from build123d import *

# Parameters (mm, degrees)
F1_DEPTH = 20
F2_R     = 5
F4_DEPTH = 8
F5_R     = 5
F6_DEPTH = 8


with BuildPart() as f1:
    # F0 (on Front) → F1 (new body, symmetric)
    with BuildSketch(Plane.XZ):
        with BuildLine():
            Line((-40, -35), (-32, -35))
            Line((-32, -35), (-32, 22))
            ThreePointArc((-32, 22), (-30.535534, 25.535534), (-27, 27))
            Line((-27, 27), (40, 27))
            Line((40, 27), (40, 35))
            Line((40, 35), (-27, 35))
            ThreePointArc((-27, 35), (-36.192388, 31.192388), (-40, 22))
            Line((-40, 22), (-40, -35))
        make_face()
    extrude(amount=F1_DEPTH, both=True)

    # F2
    f2_edges = [f1.edges().sort_by_distance(p)[0] for p in [
        (40, -20, 31),
        (40, 20, 31),
        (-36, -20, -35),
        (-36, 20, -35),
    ]]
    fillet(f2_edges, radius=F2_R)

    # F3 (on face) → F4 (cut, through all)
    with BuildSketch(Plane.XY.offset(35)):
        with BuildLine():
            Line((8, -4), (20, -4))
            ThreePointArc((20, -4), (24, 0), (20, 4))
            Line((20, 4), (8, 4))
            ThreePointArc((8, 4), (4, 0), (8, -4))
        make_face()
    extrude(amount=-F4_DEPTH, mode=Mode.SUBTRACT)

    # F5 (on face) → F6 (cut, through all)
    with BuildSketch(Plane.YZ.offset(-32)):
        with Locations((0, -20)):
            Circle(F5_R)
        with Locations((0, 5)):
            Circle(F5_R)
    extrude(amount=-F6_DEPTH, mode=Mode.SUBTRACT)


solid = f1.part
CAD build for the part. Positions are in the model's coordinates, mm. A direction names the side the tool comes from. Give positions to 0.01 mm unless a question says otherwise; leave off trailing zeros. Loops run counter-clockwise (first coordinate to the right, second up) from the corner with the lowest first, then second, coordinate; pieces in that order, holes last. Notation, with made-up numbers: M 54.25,-18 L 104.25,-18 A17 cw 104.25,-5 Z; hole C 43.25,3 d4. An arc over 180 degrees is marked long. Answer in a Markdown table with one row per item. Add a question column.
Item 1: Probe probe 1 along Y at (x, z) = (19, 28.5); probe 2 along Z at (x, y) = (-35, -2); probe 3 along Z at (x, y) = (-38, 0). List the from-to ranges inside material, lowest first.
Item 2: Band-saw the part on B-B on y = 0. Give the cut face in (x, z).
Item 3: Band-saw the part on D-D on z = 28. Give the cut face in (x, y).
Item 4: Tool access for faces 4 (the face through (-32, 0, -7)), 5 (the face through (14, -4, 31)), 6 (the face through (-36, -18, -34)): list every direction of +Z, -Z, +X, -X, +Y, -Y with a clear straight run to the whole face (end or side of a thin tool).
Item 5: Band-saw the part on A-A on x = 15.5. Give the cut face in (y, z), then the cut area to 3 significant figures.
Item 6: Drop flat-ended pins along their axis: P1, Ø1.5, axis at x = 21, y = 7, coming from the -Z side; P2, Ø12, axis at y = -0.5, z = 1, coming from the +X side. Give the stop position or say it passes through.
Item 7: Mould opens along Y. For faces 1 (the face through (-35.94, -1.08, 0.12)), 2 (the face through (39, 18, 31)), 3 (the face through (-36.091, -0.28, 31.293)) say: +Y half, -Y half, draft (parallel to the pull), parting line (faces both ways), or undercut.
Item 8: Band-saw the part on C-C on z = -20. Give the cut face in (x, y), then the cut area to 3 significant figures.
Reply:
| question | item | result |
|---|---|---|
| 1 | probe 1 | y = -20 to -4, 4 to 20 |
| 1 | probe 2 | z = -35 to -24.58, -15.42 to 0.42, 9.58 to 32.25 |
| 1 | probe 3 | z = -35 to -25, -15 to 0, 10 to 28.93 |
| 2 | outline | M -40,-35 L -32,-35 L -32,-25 L -40,-25 Z; M -40,-15 L -32,-15 L -32,0 L -40,0 Z; M -40,10 L -32,10 L -32,22 A5 cw -27,27 L 4,27 L 4,35 L -27,35 A13 ccw -40,22 Z; M 24,27 L 40,27 L 40,35 L 24,35 Z |
| 3 | outline | M -38.53,-20 L 35,-20 A5 ccw 40,-15 L 40,15 A5 ccw 35,20 L -38.53,20 Z; hole M 8,-4 L 20,-4 A4 ccw 20,4 L 8,4 A4 ccw Z |
| 4 | face 4 | -Z, +X, +Y, -Y |
| 4 | face 5 | +Z, -Z |
| 4 | face 6 | -Z, +X, -X, -Y |
| 5 | outline | M -20,27 L -4,27 L -4,35 L -20,35 Z; M 4,27 L 20,27 L 20,35 L 4,35 Z |
| 5 | area | 256 mm^2 |
| 6 | P1 | stops at z = 27 |
| 6 | P2 | stops at x = -32 |
| 7 | face 1 | undercut |
| 7 | face 2 | +Y half |
| 7 | face 3 | draft |
| 8 | outline | M -40,-20 L -32,-20 L -32,-5 L -40,-5 Z; M -40,5 L -32,5 L -32,20 L -40,20 Z |
| 8 | area | 240 mm^2 |
